Read the model definition and answer for the solid it produces. Units are mm, in the model's axes. A direction names the side the tool comes from. Round coordinates to 2 decimals unless told otherwise and drop trailing zeros. Order: outer loops, then holes, each group sorted by start corner. A loop starts at its lowest first (then second) coordinate and runs counter-clockwise, first axis right, second up. Notation, with made-up numbers: (9, 17.5) - (20, 17.5) arc R11 cw to (20, 29.5) - close; hole circle Ø11 at (63, 77). An arc over 180 degrees is marked (long way). Answer as a JSON object with one key per item and string values. Group by question number.
Q1. A tool of negligible diameter and unlimited length cuts with its end or side. For faces 1 (the flat face through (0, -19, 16)), 2 (the flat face through (38, -12.7, 16)), 3 (the flat face through (38, -25.4, 16)), from which of +Z, -Z, +X, -X, +Y, -Y can it reach the whole face along a straight path? Write none if from no direction.
Q2. A cutting plane is placed at D-D on x = 39. Determine the outline of the cut face in (y, z).
Q3. A cutting plane is placed at B-B on x = 23.5. Determine the outline of the cut face in (y, z) (3 decimals), and give its area (3 significant figures).
Q4. A cutting plane is placed at A-A on z = 23.5. Determine the outline of the cut face in (x, y).
Q5. A cutting plane is placed at C-C on y = -4. Determine the outline of the cut face in (x, z) (3 decimals), and give its area (3 significant figures).
Q6. Consider line 1 (Y direction, x = 32, z = 2); line 2 (Y direction, x = 28, z = 7.5); line 3 (X direction, y = -23, z = 21). Determine where each line is inside the solid, lowest interval first.
Q7. Given pin 1 Ø10 at (y, z) = (-6.5, 12) entering from +X; pin 2 Ø6 at (x, z) = (49.5, 9) entering from -Y; pin 3 Ø2 at (y, z) = (-30, 6.5) entering from +X, each flat-ended and moving along its own axis, determine where each tip first touches the part or whether it passes through.
```python
from build123d import *

# Parameters (mm, degrees)
F0_W     = 57.15
F0_H     = 31.75
F1_DEPTH = 38.1
F3_DEPTH = 12.7
F5_DEPTH = 25.4
F7_DEPTH = 12.7


with BuildPart() as f1:
    # F0 (on Front) → F1 (new body)
    with BuildSketch(Plane.XZ):
        with Locations((28.575, 15.875)):
            Rectangle(F0_W, F0_H)
    extrude(amount=F1_DEPTH)

    # F2 (on face) → F3 (cut)
    with BuildSketch(Plane.XZ.offset(38.1)):
        Polygon((57.15, 31.75), (19.05, 31.75), (31.75, 0), (57.15, 0), align=None)
    extrude(amount=-F3_DEPTH, mode=Mode.SUBTRACT)

    # F4 (on face) → F5 (cut)
    with BuildSketch(Plane.XZ.offset(25.4)):
        Polygon((57.15, 31.75), (44.45, 31.75), (57.15, 0), align=None)
    extrude(amount=-F5_DEPTH, mode=Mode.SUBTRACT)

    # F6 (on face) → F7 (cut)
    with BuildSketch(Plane(origin=(0, 0, 0), x_dir=(-1, 0, 0), z_dir=(0, 1, 0))):
        Polygon((-28.575, 0), (-18.325109, 31.75), (-44.45, 31.75), (-57.15, 0), align=None)
    extrude(amount=-F7_DEPTH, mode=Mode.SUBTRACT)


solid = f1.part
```
Result set:
{
 "1": {"face 1": "+Z, -Z, -X, +Y, -Y", "face 2": "+Z, +X, +Y", "face 3": "+Z, +X, -Y"},
 "2": {"outline": "(-25.4, 0) - (-12.7, 0) - (-12.7, 31.75) - (-25.4, 31.75) - close"},
 "3": {"outline": "(-38.1, 0) - (0, 0) - (0, 15.72) - (-12.7, 15.72) - (-12.7, 31.75) - (-25.4, 31.75) - (-25.4, 20.625) - (-38.1, 20.625) - close", "area": "865 mm²"},
 "4": {"outline": "(0, -38.1) - (22.35, -38.1) - (22.35, -25.4) - (47.75, -25.4) - (47.75, -12.7) - (20.99, -12.7) - (20.99, 0) - (0, 0) - close"},
 "5": {"outline": "(0, 0) - (28.575, 0) - (18.325, 31.75) - (0, 31.75) - close", "area": "745 mm²"},
 "6": {"line 1": "y = -25.4 to -12.7", "line 2": "y = -38.1 to -12.7", "line 3": "x = 0 to 48.75"},
 "7": {"pin 1": "stops at x = 26.32", "pin 2": "stops at y = -25.4", "pin 3": "stops at x = 29.55"}
}
